Autodesk Inventor part; units mm, degrees
ref_plane "YZ Plane" through (0, 0, 0) normal (1, 0, 0) x (0, 1, 0)
ref_plane "XZ Plane" through (0, 0, 0) normal (0, 1, 0) x (-1, 0, 0)
ref_plane "XY Plane" through (0, 0, 0) normal (0, 0, 1) x (1, 0, 0)
sketch "Sketch1" plane through (0, 0, 0) normal (0, 1, 0) x (-1, 0, 0)
  line L0 (10.4, 10.4) -> (-10.4, 10.4)
  line L1 (-10.4, 10.4) -> (-10.4, -10.4)
  line L2 (-10.4, -10.4) -> (10.4, -10.4)
  line L3 (10.4, -10.4) -> (10.4, 10.4)
  line L4 (10.4, 10.4) -> (-10.4, -10.4) construction
  line L5 (-10.4, 10.4) -> (10.4, -10.4) construction
  line L6 (7.5, 7.5) -> (-7.5, 7.5) construction
  line L7 (-7.5, 7.5) -> (-7.5, -7.5) construction
  line L8 (-7.5, -7.5) -> (7.5, -7.5) construction
  line L9 (7.5, -7.5) -> (7.5, 7.5) construction
  line L10 (7.5, 7.5) -> (-7.5, -7.5) construction
  line L11 (-7.5, 7.5) -> (7.5, -7.5) construction
  circle A0 centre (7.5, -7.5) radius 1.5
  circle A1 centre (-7.5, -7.5) radius 1.5
  circle A2 centre (7.5, 7.5) radius 1.5
  circle A3 centre (-7.5, 7.5) radius 1.5
  point P0 (0, 0)
  dimension "d0" = 20.8
  dimension "d1" = 20.8
  dimension "d2" = 15
  dimension "d3" = 15
  dimension "d4" = 3
  dimension "d7" = 15
  dimension "d10" = 15
extrude "Extrusion1" add sketch "Sketch1" along normal blind 1.5
sketch "Sketch2" plane through (0, 1.5, 0) normal (0, 1, 0) x (1, 0, 0)
  line L0 (10.4, 10.4) -> (-10.4, 10.4)
  line L1 (0, 10.4) -> (0, -10.4) construction
  line L2 (-10.4, -10.4) -> (10.4, -10.4)
  line L3 (-5.22, 10.3) -> (5.22, 10.3)
  line L4 (5.22, 10.3) -> (5.22, 7.85)
  line L5 (5.22, 7.85) -> (-5.22, 7.85)
  line L6 (-5.22, 7.85) -> (-5.22, 10.3)
  line L7 (-5.22, 10.3) -> (5.22, 7.85) construction
  line L8 (5.22, 10.3) -> (-5.22, 7.85) construction
  line L9 (-10.4, 10.4) -> (-10.4, -10.4)
  line L10 (-10.4, 0) -> (10.4, 0) construction
  line L11 (10.4, -10.4) -> (10.4, 10.4)
  line L12 (-5.22, -10.3) -> (5.22, -10.3)
  line L13 (5.22, -10.3) -> (5.22, -7.85)
  line L14 (5.22, -7.85) -> (-5.22, -7.85)
  line L15 (-5.22, -7.85) -> (-5.22, -10.3)
  line L16 (-5.22, -10.3) -> (5.22, -7.85) construction
  line L17 (5.22, -10.3) -> (-5.22, -7.85) construction
  point P0 (0, 0)
  point P1 (0, 9.075)
  point P2 (0, -9.075)
  dimension "d15" = 10.44
  dimension "d16" = 2.45
  dimension "d17" = 0.1
extrude "Extrusion2" add sketch "Sketch2" along normal blind 2.5 contours L3 L4 L5 L6 | L15 L14 L13 L12
equation "\"d7\" = d2"
equation "\"d10\" = d2"
properties part number "H3LIS331DL"
Geometry check sheet. Reference: the model listing, model coordinates, mm. A direction names the side the tool comes from. Give positions to 0.01 mm unless a question says otherwise; leave off trailing zeros. Order: outer loops, then holes, each group sorted by start corner. A loop starts at its lowest first (then second) coordinate and runs counter-clockwise, first axis right, second up. Notation, with made-up numbers: M 87.25,-39 L 127.25,-39 A22 ccw 127.25,-13 Z; hole C 59,-2 d11. An arc over 180 degrees is marked long. Use a Markdown table: item, result.
Item 1: Section check A-A (x = 7.5). Record the cut outline in (y, z).
Answers follow:
| item | result |
|---|---|
| outline | M 0,-10.4 L 1.5,-10.4 L 1.5,-9 L 0,-9 Z; M 0,-6 L 1.5,-6 L 1.5,6 L 0,6 Z; M 0,9 L 1.5,9 L 1.5,10.4 L 0,10.4 Z |
Item 2: Depth check by flat-ended pin: P1, Ø2.5, axis at x = 7.5, z = -7.5, coming from the +Y side; P2, Ø0.8, axis at x = 1.5, y = 2.5, coming from the +Z side; P3, Ø6, axis at x = 7.5, z = -3.5, coming from the +Y side; P4, Ø1.2, axis at y = 2.5, z = 9.5, coming from the +X side. Enter the tip coordinate at first touch or a pass-through.
Answers follow:
| item | result |
|---|---|
| P1 | passes through |
| P2 | stops at z = 10.3 |
| P3 | stops at y = 1.5 |
| P4 | stops at x = 5.22 |
Item 3: Section check D-D (x = -1). Record the cut outline in (y, z), and give its area (4 significant figures).
Answers follow:
| item | result |
|---|---|
| outline | M 0,-10.4 L 1.5,-10.4 L 1.5,-10.3 L 4,-10.3 L 4,-7.85 L 1.5,-7.85 L 1.5,7.85 L 4,7.85 L 4,10.3 L 1.5,10.3 L 1.5,10.4 L 0,10.4 Z |
| area | 43.45 mm2 |
Item 4: Material ranges on line 1 along Z through (x, y) = (7.5, 0.45); line 2 along Z through (x, y) = (-4.5, 3.65); line 3 along Z through (x, y) = (8.5, 0.95), recorded low to high.
Answers follow:
| item | result |
|---|---|
| line 1 | z = -10.4 to -9, -6 to 6, 9 to 10.4 |
| line 2 | z = -10.3 to -7.85, 7.85 to 10.3 |
| line 3 | z = -10.4 to -8.62, -6.38 to 6.38, 8.62 to 10.4 |
Item 5: Section check B-B (z = 7.5). Record the cut outline in (x, y).
Answers follow:
| item | result |
|---|---|
| outline | M -10.4,0 L -9,0 L -9,1.5 L -10.4,1.5 Z; M -6,0 L 6,0 L 6,1.5 L -6,1.5 Z; M 9,0 L 10.4,0 L 10.4,1.5 L 9,1.5 Z |
Item 6: Section check C-C (y = 2.55). Record the cut outline in (x, z), and give its area (3 significant figures).
Answers follow:
| item | result |
|---|---|
| outline | M -5.22,-10.3 L 5.22,-10.3 L 5.22,-7.85 L -5.22,-7.85 Z; M -5.22,7.85 L 5.22,7.85 L 5.22,10.3 L -5.22,10.3 Z |
| area | 51.2 mm2 |
Item 7: Draft check along Z on faces 5 (the cylindrical face through (8.7, 0.7, -6.6)), 6 (the flat face through (0, 0, 0)), 7 (the flat face through (0, 1, -10.4)). Enter one of: +Z half, -Z half, draft (parallel to the pull), parting line (faces both ways), or undercut.
Answers follow:
| item | result |
|---|---|
| face 5 | undercut |
| face 6 | draft |
| face 7 | -Z half |
Item 8: Tool access check on faces 1 (the flat face through (0, 3, -10.3)), 2 (the flat face through (5.22, 3, -9)), 3 (the flat face through (0, 3, 7.85)), 4 (the flat face through (0, 3, 10.3)). Record the directions out of +Z, -Z, +X, -X, +Y, -Y that give a thin tool (end or side, any length) a straight path to the whole face; none if there is none.
Answers follow:
| item | result |
|---|---|
| face 1 | -Z, +X, -X, +Y |
| face 2 | +Z, -Z, +X, +Y |
| face 3 | +X, -X, +Y |
| face 4 | +Z, +X, -X, +Y |
